from build123d import *

# Parameters (mm, degrees)
RESSALTO_EXTRUS_O1_DEPTH = 1.2
ESBO_O2_W                = 0.6
ESBO_O2_H                = 16
RESSALTO_EXTRUS_O2_DEPTH = 2.1
CHANFRO1_SIZE            = 1.2
CHANFRO1_SIZE2           = 0.484831471
RESSALTO_EXTRUS_O3_DEPTH = 0.6


with BuildPart() as part:
    # Esboço1 → Ressalto-extrusão1 (new body)
    with BuildSketch(Plane(origin=(0, 0, 0), x_dir=(1, 0, 0), z_dir=(0, 1, 0))):
        Polygon((2, 8.2), (2, 11.2), (-0.9, 11.2), (-0.9, 6.6), (-2, 5.654746766), (-2, -5.654746766), (-0.9, -6.6), (-0.9, -11.2), (2, -11.2), (2, -8.2), (1, -8.2), (1, 8.2), align=None)
    extrude(amount=RESSALTO_EXTRUS_O1_DEPTH)

    # Esboço2 → Ressalto-extrusão2 (add)
    with BuildSketch(Plane.XZ):
        with Locations((0.7, 0)):
            Rectangle(ESBO_O2_W, ESBO_O2_H)
    extrude(amount=RESSALTO_EXTRUS_O2_DEPTH)

    # Chanfro1
    chanfro1_edges = [part.edges().sort_by_distance(p)[0] for p in [
        (1, -2.1, 0),
    ]]
    chanfro1_side = [part.faces().sort_by_distance(p)[0] for p in [
        (1, -0.440540541, 0),
    ]]
    chamfer(chanfro1_edges, length=CHANFRO1_SIZE, length2=CHANFRO1_SIZE2, reference=chanfro1_side[0])

    # Esboço3 → Ressalto-extrusão3 (add)
    with BuildSketch(Plane.ZY.offset(-0.4)):
        with BuildLine():
            Line((-8.25, -1.5), (-8.5, -1.5))
            ThreePointArc((-8.5, -1.5), (-8.853553391, -1.646446609), (-9, -2))
            Line((-9, -2), (-9, -3.8))
            ThreePointArc((-9, -3.8), (-9.117157288, -4.082842712), (-9.4, -4.2))
            Line((-9.4, -4.2), (-9.6, -4.2))
            ThreePointArc((-9.6, -4.2), (-9.882842712, -4.082842712), (-10, -3.8))
            Line((-10, -3.8), (-10, -3.4))
            Line((-10, -3.4), (-9.65, -3.4))
            Line((-9.65, -3.4), (-9.65, -2.55))
            Line((-9.65, -2.55), (-9.8, -2.2))
            Line((-9.8, -2.2), (-9.65, -1.5))
            Line((-9.65, -1.5), (-9.65, -0.7))
            Line((-9.65, -0.7), (-9.85, -0.5))
            Line((-9.85, -0.5), (-9.85, -0.3))
            Line((-9.85, -0.3), (-9.65, 0))
            Line((-9.65, 0), (-8, 0))
            Line((-8, 0), (-8, -1.75))
            ThreePointArc((-8, -1.75), (-8.073223305, -1.573223305), (-8.25, -1.5))
        make_face()
    ressalto_extrus_o3 = extrude(amount=-RESSALTO_EXTRUS_O3_DEPTH)

    # Espelhar1: Ressalto-extrusão3 across plane
    add(ressalto_extrus_o3.mirror(Plane.XY))


solid = part.part
Geometry: final body of the model. Coordinates: model frame, mm. A direction names the side the tool comes from. Round coordinates to 2 decimals unless told otherwise and drop trailing zeros. Write each loop counter-clockwise with the first axis right and the second up, starting at its lowest first coordinate (ties: lowest second). Pieces come first, ordered by that corner, then holes. Notation, with made-up numbers: M 72.5,13 L 102.5,13 A36 cw 102.5,50 Z; hole C 2.5,67.5 d8. An arc over 180 degrees is marked long. Write item = value, one per line.
Item 1: Access query for faces 1 (the face through (-0.9, 1, 9)), 2 (the face through (1.5, 0.6, 8.2)), 3 (the face through (0.4, -1, -2)). Directions: +Z, -Z, +X, -X, +Y, -Y. A direction counts if a zero-diameter tool reaches every point of the face in a straight line with its end or side. Return the directions, or none.
Findings:
face_1 = +Z, -X, +Y, -Y
face_2 = +X, +Y, -Y
face_3 = +Z, -Z, -X, -Y
Item 2: Section query D-D on x = -0.3. Return loops of the section in (y, z), then the cut area to 3 significant figures.
Findings:
outline = M 0,-11.2 L 1.2,-11.2 L 1.2,11.2 L 0,11.2 Z
area = 26.9 mm^2
Item 3: Section query A-A on x = 1.25. Return loops of the section in (y, z), then the cut area to 3 significant figures.
Findings:
outline = M 0,-11.2 L 1.2,-11.2 L 1.2,-8.2 L 0,-8.2 Z; M 0,8.2 L 1.2,8.2 L 1.2,11.2 L 0,11.2 Z
area = 7.20 mm^2
Item 4: Pull-direction query (Z, two-part tool) for faces 4 (the face through (1, 1, 11.2)), 5 (the face through (0.754, -1.508, -0.112)), 6 (the face through (-0.9, 1, -9)), 7 (the face through (1, 1, -11.2)); classes: pulls with the +Z half, pulls with the -Z half, needs draft (parallel to the pull), parting line crosses it, or undercut.
Findings:
face_4 = pulls with the +Z half
face_5 = undercut
face_6 = needs draft
face_7 = pulls with the -Z half
Item 5: Material intervals for line 1 along Z through (x, y) = (1.15, 0.6); line 2 along Z through (x, y) = (0.7, -0.75); line 3 along X through (y, z) = (0.8, -8), sorted ascending. Write a range as [from, to].
Findings:
line_1 = [-11.2, -8.2], [8.2, 11.2]
line_2 = [-9.65, 9.65]
line_3 = [-0.9, 1]
Item 6: Section query B-B on y = -2.95. Return loops of the section in (x, z), then the cut area to 3 significant figures.
Findings:
outline = M 0.4,-9.65 L 1,-9.65 L 1,-9 L 0.4,-9 Z; M 0.4,9 L 1,9 L 1,9.65 L 0.4,9.65 Z
area = 0.780 mm^2
Item 7: Section query C-C on z = -7. Return loops of the section in (x, y), then the cut area to 3 significant figures.
Findings:
outline = M -0.9,0 L 0.4,0 L 0.4,-2.1 L 0.52,-2.1 L 1,-0.9 L 1,1.2 L -0.9,1.2 Z
area = 3.25 mm^2
Item 8: Pin query (flat end, axial travel): P1, Ø1.5, axis at y = -2.5, z = 4.5, coming from the +X side; P2, Ø0.7, axis at x = 0.5, y = -3, coming from the -Z side; P3, Ø0.7, axis at x = 0.5, y = -3, coming from the +Z side. Return the tip coordinate at first contact, or that it passes through.
Findings:
P1 = 0.66
P2 = -9.65
P3 = 9.65
